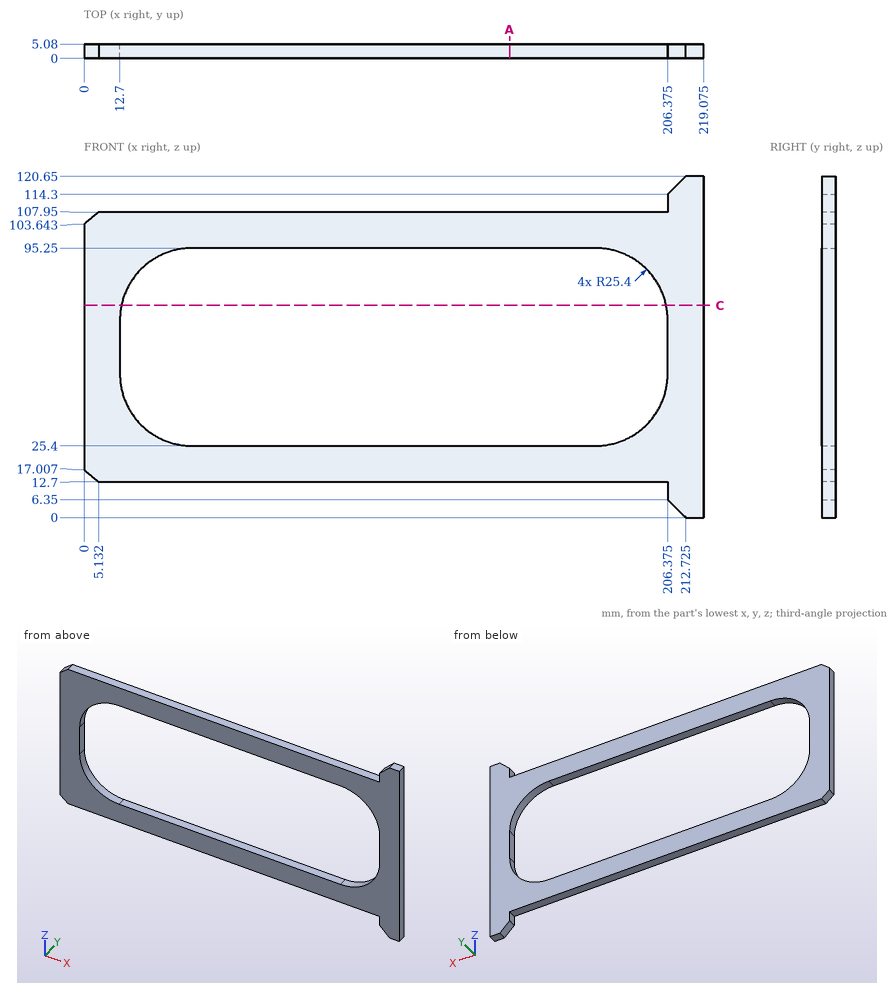
Check sheet for the drawn part. Datum: minimum x, y, z corner. Units: mm. Coordinates: 2 decimals unless noted, no trailing zeros. Loops run counter-clockwise (first coordinate to the right, second up) from the corner with the lowest first, then second, coordinate; pieces in that order, holes last. Notation, with made-up numbers: (2.5, 18) -> (58.5, 18) arc R6 cw to (58.5, 28) -> close; hole circle Ø4 at (-18, -3.75). An arc over 180 degrees is marked (long way). Answer as a JSON object with one key per item and string values. Group by question number.
Item 1: Scan lines: probe 1 along Z at (x, y) = (152.5, 4.85); probe 2 along X at (y, z) = (1.3, 56.5) (1 decimal); probe 3 along X at (y, z) = (0.35, 45.5) (1 decimal). Record each from-to range of solid material in increasing order.
Item 2: Depth check by flat-ended pin: pin 1 (1.5 mm diameter, centred on x = 100, y = 3.5, fed in from -Z). Enter the tip coordinate at first touch or a pass-through.
Item 3: Sectioned sample at C-C on z = 75. Record the boundary of the cut face in (x, y) (1 decimal), plus the area to 3 significant figures.
Item 4: Sectioned sample at A-A on x = 150.5. Record the boundary of the cut face in (y, z), plus the area to 3 significant figures.
Evaluation:
{
 "1": {"probe 1": "z = 12.7 to 25.4, 95.25 to 107.95", "probe 2": "x = 0 to 12.7, 206.4 to 219.1", "probe 3": "x = 0 to 13.3, 205.8 to 219.1"},
 "2": {"pin 1": "stops at z = 12.7"},
 "3": {"outline": "(0, 0) -> (13.2, 0) -> (13.2, 5.1) -> (0, 5.1) -> close; (205.8, 0) -> (219.1, 0) -> (219.1, 5.1) -> (205.8, 5.1) -> close", "area": "134 mm²"},
 "4": {"outline": "(0, 12.7) -> (5.08, 12.7) -> (5.08, 25.4) -> (0, 25.4) -> close; (0, 95.25) -> (5.08, 95.25) -> (5.08, 107.95) -> (0, 107.95) -> close", "area": "129 mm²"}
}
